```python
from build123d import *

# Parameters (mm, degrees)
F0_W     = 22.86
F0_H     = 203.2
F1_DEPTH = 25.4


# Not quite as in the source:
# - ends of sketch curves that miss each other by under 0.0002 mm in the source are joined


with BuildPart() as f1:
    # F0 (on Front) → F1 (new body)
    with BuildSketch(Plane.XZ):
        with Locations((-0.3399215189, 11.8189063548)):
            Rectangle(F0_W, F0_H)
        with BuildLine():
            Line((7.5848784811, -7.2097627448), (-2.2264276225, -37.4049924117))
            ThreePointArc((-2.2264276225, -37.4049924117), (-6.2271781929, -39.4434341876), (-8.2656199687, -35.4426836172))
            Line((-8.2656199687, -35.4426836172), (1.5459240038, -5.2467218859))
            ThreePointArc((1.5459240926, -5.2467219148), (5.5470406879, -3.2083990956), (7.5848784811, -7.2097627448))
        make_face(mode=Mode.SUBTRACT)
        with BuildLine():
            Line((7.5848784811, -42.1355889051), (-2.2258696668, -72.3299669673))
            ThreePointArc((-2.2258696668, -72.3299669673), (-6.2266030631, -74.3684424494), (-8.2650785452, -70.367709053))
            Line((-8.2650785452, -70.367709053), (1.5462110262, -40.1716646606))
            ThreePointArc((1.5462110262, -40.1716646606), (5.5477780101, -38.1334601546), (7.5848784811, -42.1355889051))
        make_face(mode=Mode.SUBTRACT)
        with BuildLine():
            Line((7.5848784811, 27.7160793915), (-2.2264110515, -2.4799669119))
            ThreePointArc((-2.2264110515, -2.4799669119), (-6.2271444076, -4.5184424731), (-8.2656199687, -0.517709117))
            Line((-8.2656199687, -0.517709117), (1.5456690059, 29.6783354693))
            ThreePointArc((1.5456690059, 29.6783354693), (5.5464015034, 31.7168113094), (7.5848784811, 27.7160793915))
        make_face(mode=Mode.SUBTRACT)
        with BuildLine():
            Line((7.5848784811, 97.5660773977), (-2.2264110903, 67.3700330053))
            ThreePointArc((-2.2264110903, 67.3700330053), (-6.2271444866, 65.3315575232), (-8.2656199687, 69.3322909196))
            Line((-8.2656199687, 69.3322909196), (1.5456696027, 99.528335312))
            ThreePointArc((1.5456696027, 99.528335312), (5.546402999, 101.5668107941), (7.5848784811, 97.5660773977))
        make_face(mode=Mode.SUBTRACT)
        with BuildLine():
            Line((7.5848784811, 62.6383122648), (-2.2255126404, 32.4450330169))
            ThreePointArc((-2.2255126404, 32.4450330169), (-6.2262460368, 30.4065575348), (-8.2647215189, 34.4072909311))
            Line((-8.2647215189, 34.4072909311), (1.5465680525, 64.6033353235))
            ThreePointArc((1.5465680525, 64.6033353235), (5.5486851845, 66.6413608527), (7.5848784811, 62.6383122648))
        make_face(mode=Mode.SUBTRACT)
    extrude(amount=F1_DEPTH)


solid = f1.part
```
CAD build for the part. Positions are in the model's coordinates, mm. A direction names the side the tool comes from. Coordinates: 2 decimals unless noted, no trailing zeros. Write each loop counter-clockwise with the first axis right and the second up, starting at its lowest first coordinate (ties: lowest second). Pieces come first, ordered by that corner, then holes. Notation, with made-up numbers: (-7, 58.5) -> (7, 58.5) arc R25 ccw to (7, 77.5) -> close; hole circle Ø10 at (-26, -37.5). An arc over 180 degrees is marked (long way). Use CSV: the item, a comma, the result in double quotes. Start each with the question number.
Item 1: Drop a flat-ended pin along its axis: P1, Ø5, axis at x = 5.5, z = 26, coming from the -Y side. Give the stop position or say it passes through.
Item 2: Wall check: probe 1 along X at (y, z) = (-11, 32.5); probe 2 along X at (y, z) = (-11.75, 31); probe 3 along X at (y, z) = (-21, 14.5). Give the ranges that are in metal, low to high.
Item 3: Band-saw the part on A-A, the plane y = -8.5. Write the cut outline in (x, z) (3 decimals).
Item 4: Two-plate mould, pull along Z, no slides. Class faces 1 (the flat face through (0, -13, -89.781)), 2 (the flat face through (-6, 0, 13)), 3 (the flat face through (2.75, -12.52, 12.83)): +Z half, -Z half, draft (parallel to the pull), parting line (faces both ways), or undercut.
Item 5: Band-saw the part on C-C, the plane z = -26. Write the cut outline in (x, y), plus the area to 3 significant figures.
Item 6: Band-saw the part on B-B, the plane z = -67. Write the cut outline in (x, y), plus the area to 3 significant figures.
Item 7: Tool access for faces 4 (the flat face through (-11.77, -13, 10)), 5 (the flat face through (-3.428, -12.522, -55.481)): list every direction of +Z, -Z, +X, -X, +Y, -Y with a clear straight run to the whole face (end or side of a thin tool).
Response values:
1,P1,"stops at y = -25.4"
2,probe 1,"x = -11.77 to -8.28, -2.21 to 11.09"
2,probe 2,"x = -11.77 to -7.29, -3.2 to 2.38, 6.75 to 11.09"
2,probe 3,"x = -11.77 to -3.39, 3.29 to 11.09"
3,outline,"(-11.77, -89.781) -> (11.09, -89.781) -> (11.09, 113.419) -> (-11.77, 113.419) -> close; hole (-8.266, -35.443) arc R3.175 ccw to (-2.226, -37.405) -> (7.585, -7.21) arc R3.175 ccw to (1.546, -5.247) -> close; hole (-8.266, -0.518) arc R3.175 ccw to (-2.226, -2.48) -> (7.585, 27.716) arc R3.175 ccw to (1.546, 29.678) -> close; hole (-8.266, 69.332) arc R3.175 ccw to (-2.226, 67.37) -> (7.585, 97.566) arc R3.175 ccw to (1.546, 99.528) -> close; hole (-8.265, -70.368) arc R3.175 ccw to (-2.226, -72.33) -> (7.585, -42.136) arc R3.175 ccw to (1.546, -40.172) -> close; hole (-8.265, 34.407) arc R3.175 ccw to (-2.226, 32.445) -> (7.585, 62.638) arc R3.175 ccw to (1.547, 64.603) -> close"
4,face 1,"-Z half"
4,face 2,"draft"
4,face 3,"undercut"
5,outline,"(-11.77, -25.4) -> (-5.2, -25.4) -> (-5.2, 0) -> (-11.77, 0) -> close; (1.48, -25.4) -> (11.09, -25.4) -> (11.09, 0) -> (1.48, 0) -> close"
5,area,"411 mm2"
6,outline,"(-11.77, -25.4) -> (-7.17, -25.4) -> (-7.17, 0) -> (-11.77, 0) -> close; (-0.49, -25.4) -> (11.09, -25.4) -> (11.09, 0) -> (-0.49, 0) -> close"
6,area,"411 mm2"
7,face 4,"+Z, -Z, -X, +Y, -Y"
7,face 5,"+Y, -Y"
